Input: part model. Units: mm. Frame: model coordinates. Face numbers are marked on the shaded views. A direction names the side the tool comes from. Give positions to 0.01 mm unless a question says otherwise; leave off trailing zeros. Loops run counter-clockwise (first coordinate to the right, second up) from the corner with the lowest first, then second, coordinate; pieces in that order, holes last. Notation, with made-up numbers: (-3.5, 53.5) - (7.5, 53.5) arc R19 cw to (7.5, 83.5) - close; hole circle Ø6 at (68, -22.75). An arc over 180 degrees is marked (long way). Answer as a JSON object with one key per item and string values.
from build123d import *

# Parameters (mm, degrees)
SKETCH1_R                                            = 2
BOSS_EXTRUDE1_DEPTH                                  = 5
FILLET1_R                                            = 3
SKETCH2_W                                            = 8
SKETCH2_H                                            = 10
BOSS_EXTRUDE3_DEPTH                                  = 1
CSK_FOR_M1_6_COUNTERSUNK_FLAT_HEAD_SCREW_D           = 1.8
CSK_FOR_M1_6_COUNTERSUNK_FLAT_HEAD_SCREW_DEPTH       = 30
CSK_FOR_M1_6_COUNTERSUNK_FLAT_HEAD_SCREW_CSINK_D     = 3.6
CSK_FOR_M1_6_COUNTERSUNK_FLAT_HEAD_SCREW_CSINK_ANGLE = 90
CSK_FOR_M1_6_COUNTERSUNK_FLAT_HEAD_SCREW_TIP         = 0.540774557


with BuildPart() as part:
    # Sketch1 → Boss-Extrude1 (new body)
    with BuildSketch(Plane(origin=(0, 0, 0), x_dir=(0, 0, -1), z_dir=(1, 0, 0))):
        with BuildLine():
            Line((1, 2), (18.101020514, 2))
            ThreePointArc((18.101020514, 2), (28, 3), (18.101020514, 4))
            Line((18.101020514, 4), (-1, 4))
            Line((-1, 4), (-1, 0))
            Line((-1, 0), (1, 0))
            Line((1, 0), (1, 2))
        make_face()
        with Locations((23, 3)):
            Circle(SKETCH1_R, mode=Mode.SUBTRACT)
    extrude(amount=BOSS_EXTRUDE1_DEPTH)

    # Fillet1
    # the kernel refuses this fillet: 3 mm, written as the material it adds along each edge
    with BuildSketch(Plane(origin=(0, 2, -1), x_dir=(0, 0, -1), z_dir=(1, 0, 0))) as fillet1_piece_1:
        with BuildLine():
            CenterArc((2.828427125, -3), FILLET1_R, 90, 70.528779366)
            Line((0, -2), (-0.056568542, -1.98))
            ThreePointArc((-0.056568542, -1.98), (-0.06, -1), (-0.06, 0))
            Line((-0.06, 0), (0, 0.06))
            Line((0, 0.06), (2.828427125, 0.06))
            Line((2.828427125, 0.06), (2.828427125, 0))
        make_face()
    extrude(amount=5)

    # Sketch2 → Boss-Extrude3 (add)
    with BuildSketch(Plane.XZ):
        with Locations((2.5, 0)):
            Rectangle(SKETCH2_W, SKETCH2_H)
    extrude(amount=-BOSS_EXTRUDE3_DEPTH)

    # CSK for M1.6 Countersunk Flat Head Screw1
    with Locations(Plane(origin=(0, 1, 0), x_dir=(1, 0, 0), z_dir=(0, 1, 0))):
        with Locations((2.5, -3)):
            CounterSinkHole(CSK_FOR_M1_6_COUNTERSUNK_FLAT_HEAD_SCREW_D / 2, CSK_FOR_M1_6_COUNTERSUNK_FLAT_HEAD_SCREW_CSINK_D / 2, depth=CSK_FOR_M1_6_COUNTERSUNK_FLAT_HEAD_SCREW_DEPTH, counter_sink_angle=CSK_FOR_M1_6_COUNTERSUNK_FLAT_HEAD_SCREW_CSINK_ANGLE)
            with Locations((0, 0, -(CSK_FOR_M1_6_COUNTERSUNK_FLAT_HEAD_SCREW_DEPTH + CSK_FOR_M1_6_COUNTERSUNK_FLAT_HEAD_SCREW_TIP / 2))):  # 118° drill point
                Cone(0, CSK_FOR_M1_6_COUNTERSUNK_FLAT_HEAD_SCREW_D / 2, CSK_FOR_M1_6_COUNTERSUNK_FLAT_HEAD_SCREW_TIP, mode=Mode.SUBTRACT)


solid = part.part
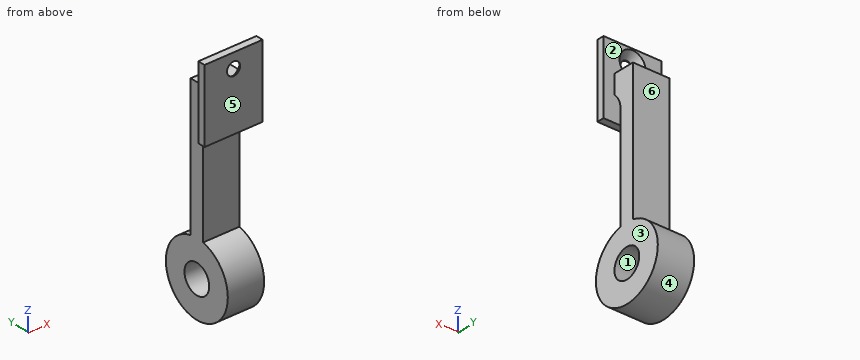
Item 1: Cut plane C-C (x = 2.5). Return loops of the section in (y, z), then the cut area to 3 significant figures.
Geometry check:
{"outline": "(0, -5) - (1, -5) - (1, -1.59) arc R3 cw to (2, -3.83) - (2, -18.1) arc R5 ccw (long way) to (4, -18.1) - (4, 1) - (1, 1) - (1, 1.2) - (0.1, 2.1) - (0, 2.1) - close; (0, 3.9) - (0.1, 3.9) - (1, 4.8) - (1, 5) - (0, 5) - close; hole circle Ø4 at (3, -23)", "area": "115 mm2"}
Item 2: Contact query for flat-ended pins moving along their axis: P1, Ø3, axis at y = 0, z = -21, coming from the +X side; P2, Ø1.5, axis at x = 2.5, y = 3, coming from the +Z side; P3, Ø1, axis at y = 3, z = -10.5, coming from the -X side; P4, Ø1.6, axis at x = 2.5, z = 3, coming from the -Y side. Output: stop coordinate, or through.
Geometry check:
{"P1": "stops at x = 5", "P2": "stops at z = 1", "P3": "stops at x = 0", "P4": "passes through"}
Item 3: Cut plane D-D (z = -23). Return loops of the section in (x, y).
Geometry check:
{"outline": "(0, -2) - (5, -2) - (5, 1) - (0, 1) - close; (0, 5) - (5, 5) - (5, 8) - (0, 8) - close"}
Item 4: Cut plane A-A (z = 3). Return loops of the section in (x, y), then the cut area to 3 significant figures.
Geometry check:
{"outline": "(-1.5, 0) - (1.6, 0) - (1.6, 0.1) - (0.7, 1) - (-1.5, 1) - close; (3.4, 0) - (6.5, 0) - (6.5, 1) - (4.3, 1) - (3.4, 0.1) - close", "area": "5.39 mm2"}
Item 5: Mould query, pull axis Z, two halves, no side actions, for the marked faces 1, 2 and 3. Classes: released by +Z, released by -Z, zero draft, split by the parting line, or undercut.
Geometry check:
{"face 1": "undercut", "face 2": "undercut", "face 3": "zero draft"}
Item 6: Access query for the marked faces 4, 5 and 6. Directions: +Z, -Z, +X, -X, +Y, -Y. A direction counts if a zero-diameter tool reaches every point of the face in a straight line with its end or side. Return the directions, or none.
Geometry check:
{"face 4": "+X, -X", "face 5": "+Z, +X, -X, -Y", "face 6": "+Z, +X, -X, +Y"}
Item 7: Cut plane B-B (y = 3). Return loops of the section in (x, z), then the cut area to 3 significant figures.
Geometry check:
{"outline": "(0, -28) - (5, -28) - (5, -25) - (0, -25) - close; (0, -21) - (5, -21) - (5, 1) - (0, 1) - close", "area": "125 mm2"}
Item 8: Material intervals for line 1 (Z direction, x = 2.5, y = 0.05); line 2 (X direction, y = 2.5, z = -10); line 3 (Y direction, x = 1.65, z = -23), sorted ascending. Write a range as [from, to].
Geometry check:
{"line 1": "z = [-27.04, -18.96], [-5, 2.1], [3.9, 5]", "line 2": "x = [0, 5]", "line 3": "y = [-2, 1], [5, 8]"}
